```python
from build123d import *

# Parameters (mm, degrees)
F0_R     = 10.5
F1_DEPTH = 1.5


with BuildPart() as f1:
    # F0 (on Top) → F1 (new body)
    with BuildSketch(Plane.XY):
        Circle(F0_R)
    extrude(amount=-F1_DEPTH)

    # F5 (on offset) → F6 section 0
    with BuildSketch(Plane.XZ.offset(-5.4)):
        Polygon((-1.75, 0), (1.75, 0), (2.75, 1.7), (-2.75, 1.7), align=None)
    # F3 (on offset) → F6 section 1
    with BuildSketch(Plane.XZ.offset(3)):
        Polygon((-1.25, 0), (1.25, 0), (2.25, 1.7), (-2.25, 1.7), align=None)
    loft()


solid = f1.part
```
Here's how the part is built. I have some questions about the finished solid (model axes, mm). A direction names the side the tool comes from. Give positions to 0.01 mm unless a question says otherwise; leave off trailing zeros. Write each loop counter-clockwise with the first axis right and the second up, starting at its lowest first coordinate (ties: lowest second). Pieces come first, ordered by that corner, then holes. Notation, with made-up numbers: (-11.5, 50) -> (5.5, 50) arc R21 ccw to (5.5, 86) -> close; hole circle Ø8 at (-1, -29.75). An arc over 180 degrees is marked (long way). Use one line per item in the form item = value.
1) Suppose I cut it at A-A (z = -0.35). Please give me the cut outline in (x, y), and give its area (3 significant figures).
Verdict:
outline = circle Ø21 at (0, 0)
area = 346 mm2
2) Suppose I cut it at B-B (x = 8). Please give me the cut outline in (y, z), and give its area (3 significant figures).
Verdict:
outline = (-6.8, -1.5) -> (6.8, -1.5) -> (6.8, 0) -> (-6.8, 0) -> close
area = 20.4 mm2
3) Suppose I cut it at C-C (y = -4.5). Please give me the cut outline in (x, z).
Verdict:
outline = (-9.49, -1.5) -> (9.49, -1.5) -> (9.49, 0) -> (-9.49, 0) -> close
4) On a 3-axis mill with a long thin cutter (end or side, diameter ignored), from which of +Z, -Z, +X, -X, +Y, -Y can I reach the whole of each face in a straight line? I mean faces 1 (the face through (0, -3, 1)), 2 (the face through (10, 3.2, -0.7)), 3 (the face through (0, 5.4, 1)). Say none if no direction works.
Verdict:
face_1 = +Z, +X, -X, -Y
face_2 = +Z, -Z
face_3 = +Z, +X, -X, +Y
5) I'm going to push flat-ended pins straight in: pin 1 (1 mm diameter, centred on x = -5, y = -2, fed in from +Z); pin 2 (0.5 mm diameter, centred on x = -0.5, z = 1, fed in from +Y); pin 3 (1 mm diameter, centred on x = -5, z = 1, fed in from +Y). Where does each tip first touch, or does it pass through?
Verdict:
pin_1 = 0
pin_2 = 5.4
pin_3 = through
6) If I drill on L1, parallel to Z at x = -2.25, y = -7.75; L2, parallel to Y at x = -1.25, z = 0.9; L3, parallel to X at y = 9.75, z = -0.4, over which ranges is the centre line in solid material (lowest first)? Write a range as [from, to].
Verdict:
L1 = [-1.5, 0]
L2 = [-3, 5.4]
L3 = [-3.9, 3.9]
